Here's how the part is built. I have some questions about the finished solid (model axes, mm). A direction names the side the tool comes from. Round coordinates to 2 decimals unless told otherwise and drop trailing zeros. Write each loop counter-clockwise with the first axis right and the second up, starting at its lowest first coordinate (ties: lowest second). Pieces come first, ordered by that corner, then holes. Notation, with made-up numbers: (29.25, 89) -> (38.25, 89) arc R25 cw to (38.25, 113) -> close; hole circle Ø6 at (-30.75, 78). An arc over 180 degrees is marked (long way). Put each result on its own line as item: value. Start each with the question number.
1. Suppose I cut it at B-B (y = -2). Please give me the cut outline in (x, z), then the cut area to 3 significant figures.
2. Suppose I cut it at D-D (x = 31). Please give me the cut outline in (y, z).
3. We'd pull the mould along X, two halves only. Please class faces 5 (the face through (75, 0, 2)), 6 (the face through (37, 0, 0)), 7 (the face through (0, 0, 2)): +X half, -X half, draft (parallel to the pull), parting line (faces both ways), or undercut.
4. Suppose I cut it at A-A (x = 70). Please give me the cut outline in (y, z).
5. Suppose I cut it at C-C (z = 2). Please give me the cut outline in (x, y), then the cut area to 3 significant figures.
6. I need wall thicknesses on probe 1 along Z at (x, y) = (38.5, -2); probe 2 along Y at (x, z) = (56.5, 5). Which ranges of each line are inside material? Lowest first, please. Write a range as from..to.
7. For pin 1 (1.5 mm diameter, centred on x = 23.5, y = 3.5, fed in from +Z); pin 2 (2 mm diameter, centred on x = 35.5, z = 4, fed in from +Y); pin 3 (0.5 mm diameter, centred on y = 0, z = 7.5, fed in from +X), each with a flat end and sliding along its axis, tell me the tip position at first contact or that it passes through.
8. Which directions (+Z, -Z, +X, -X, +Y, -Y) give clear straight access to the entire face, cutting with the end or side of a thin tool? Please do faces 1 (the face through (32, 0, 8)), 2 (the face through (37, 1, 5)), 3 (the face through (70, 0, 7)), 4 (the face through (37, -1, 4)).
```python
from build123d import *

# Parameters (mm, degrees)
PAD_DEPTH         = 75
SKETCH001_W       = 10
SKETCH001_H       = 1
POCKET_DEPTH      = 10.001
POCKET_DEPTH_BACK = -10.001


with BuildPart() as part:
    # Sketch → Pad (new body)
    with BuildSketch(Plane.YZ):
        Polygon((-10, 1), (-1, 1), (-1, 8), (1, 8), (1, 1), (10, 1), (10, 0), (-10, 0), align=None)
    extrude(amount=PAD_DEPTH)

    # Sketch001 → Pocket (cut, two sides)
    with BuildSketch(Plane.XZ) as pocket_sk:
        with Locations((70, 7.5)):
            Rectangle(SKETCH001_W, SKETCH001_H)
    extrude(amount=-POCKET_DEPTH, mode=Mode.SUBTRACT)
    extrude(pocket_sk.sketch, amount=-POCKET_DEPTH_BACK, mode=Mode.SUBTRACT)


solid = part.part
```
Verdict:
1. outline: (0, 0) -> (75, 0) -> (75, 1) -> (0, 1) -> close
1. area: 75.0 mm^2
2. outline: (-10, 0) -> (10, 0) -> (10, 1) -> (1, 1) -> (1, 8) -> (-1, 8) -> (-1, 1) -> (-10, 1) -> close
3. face 5: +X half
3. face 6: draft
3. face 7: -X half
4. outline: (-10, 0) -> (10, 0) -> (10, 1) -> (1, 1) -> (1, 7) -> (-1, 7) -> (-1, 1) -> (-10, 1) -> close
5. outline: (0, -1) -> (75, -1) -> (75, 1) -> (0, 1) -> close
5. area: 150 mm^2
6. probe 1: z = 0..1
6. probe 2: y = -1..1
7. pin 1: stops at z = 1
7. pin 2: stops at y = 1
7. pin 3: stops at x = 65
8. face 1: +Z, +X, -X, +Y, -Y
8. face 2: +Z, +X, -X, +Y
8. face 3: +Z, +X, +Y, -Y
8. face 4: +Z, +X, -X, -Y
